CAD build for the part. Positions are in the model's coordinates, mm. Round coordinates to 2 decimals unless told otherwise and drop trailing zeros. Order: outer loops, then holes, each group sorted by start corner. A loop starts at its lowest first (then second) coordinate and runs counter-clockwise, first axis right, second up. Notation, with made-up numbers: M 33.5,80.25 L 76.5,80.25 A31 cw 76.5,111.25 Z; hole C 30.5,70.5 d4. An arc over 180 degrees is marked long. Put each result on its own line as item: value.
```python
from build123d import *

# Parameters (mm, degrees)
SKETCH_1_R      = 2.25
SKETCH_1_R_2    = 1.7
SKETCH_1_R_3    = 6
SKETCH_1_R_4    = 4.75
SKETCH_1_R_5    = 5
SKETCH_1_R_6    = 1.69491354
EXTRUDE_1_DEPTH = 2


with BuildPart() as part:
    # 草图1 → 凸台-拉伸1 (new body)
    with BuildSketch(Plane(origin=(0, 0, 0), x_dir=(1, 0, 0), z_dir=(0, 1, 0))):
        Polygon((-41.878679656, -46.121320344), (42.121320344, -46.121320344), (44.23849367, -43.995861074), (44.23849367, 44.004138926), (42.249509012, 46.250010702), (-42.015698652, 46.250010702), (-44, 44), (-44, -44), align=None)
        with Locations(Location((-15.25, -15.25, 0), (0, 0, 270))):
            Circle(SKETCH_1_R, mode=Mode.SUBTRACT)
        with Locations(Location((-15.25, 15.25, 0), (0, 0, 270))):
            Circle(SKETCH_1_R, mode=Mode.SUBTRACT)
        with Locations(Location((15.25, -15.25, 0), (0, 0, 270))):
            Circle(SKETCH_1_R, mode=Mode.SUBTRACT)
        with Locations(Location((15.25, 15.25, 0), (0, 0, 270))):
            Circle(SKETCH_1_R, mode=Mode.SUBTRACT)
        with Locations(Location((-24, -33, 0), (0, 0, 270))):
            Circle(SKETCH_1_R_2, mode=Mode.SUBTRACT)
        with Locations(Location((20, 0, 0), (0, 0, 270))):
            Circle(SKETCH_1_R_3, mode=Mode.SUBTRACT)
        with Locations(Location((-20, 0, 0), (0, 0, 270))):
            Circle(SKETCH_1_R_4, mode=Mode.SUBTRACT)
        with Locations(Location((0, 26, 0), (0, 0, 270))):
            Circle(SKETCH_1_R_5, mode=Mode.SUBTRACT)
        with Locations(Location((0, -26, 0), (0, 0, 270))):
            Circle(SKETCH_1_R_5, mode=Mode.SUBTRACT)
        with Locations(Location((-30.40559154, -40.30508646, 0), (0, 0, 270))):
            Circle(SKETCH_1_R_2, mode=Mode.SUBTRACT)
        with Locations(Location((-30.40559154, 40.30508646, 0), (0, 0, 270))):
            Circle(SKETCH_1_R_2, mode=Mode.SUBTRACT)
        with Locations(Location((-40.30508646, 30.40559154, 0), (0, 0, 270))):
            Circle(SKETCH_1_R_2, mode=Mode.SUBTRACT)
        with Locations(Location((30.40559154, -40.30508646, 0), (0, 0, 270))):
            Circle(SKETCH_1_R_2, mode=Mode.SUBTRACT)
        with Locations(Location((40.30508646, -31, 0), (0, 0, 270))):
            Circle(SKETCH_1_R_6, mode=Mode.SUBTRACT)
        with Locations(Location((40.30508646, 30.40559154, 0), (0, 0, 270))):
            Circle(SKETCH_1_R_6, mode=Mode.SUBTRACT)
        with Locations(Location((30.40559154, 40.30508646, 0), (0, 0, 270))):
            Circle(SKETCH_1_R_2, mode=Mode.SUBTRACT)
        with Locations(Location((-40.30508646, -30.40559154, 0), (0, 0, 90))):
            Circle(SKETCH_1_R_2, mode=Mode.SUBTRACT)
        with Locations(Location((24, -33, 0), (0, 0, 90))):
            Circle(SKETCH_1_R_2, mode=Mode.SUBTRACT)
        with Locations(Location((24, 33, 0), (0, 0, 270))):
            Circle(SKETCH_1_R_2, mode=Mode.SUBTRACT)
        with Locations(Location((-24, 33, 0), (0, 0, 90))):
            Circle(SKETCH_1_R_2, mode=Mode.SUBTRACT)
    extrude(amount=EXTRUDE_1_DEPTH)


solid = part.part
```
Item 1: Band-saw the part on D-D on y = 0.7. State how many separate pieces and enclosed holes the cut face has, and give its area (3 significant figures).
Answers below:
separate pieces: 1
enclosed holes: 20
area: 7,630 mm²
Item 2: Band-saw the part on B-B on x = 20. Give the cut face in (y, z).
Answers below:
outline: M 0,-46.25 L 2,-46.25 L 2,-6 L 0,-6 Z; M 0,6 L 2,6 L 2,46.12 L 0,46.12 Z
Item 3: Mould opens along Z. For faces 1 (the cylindrical face through (21.802, 0.986, 5.723)), 2 (the flat face through (43.17, 0.99, 45.07)), 3 (the flat face through (-42.994, 0.986, -45.141)), 4 (the cylindrical face through (25.433, 0.986, -32.086)) say: pulls with the +Z half, pulls with the -Z half, needs draft (parallel to the pull), parting line crosses it, or undercut.
Answers below:
face 1: undercut
face 2: pulls with the +Z half
face 3: pulls with the -Z half
face 4: undercut
Item 4: Band-saw the part on A-A on x = 0. Give the cut face in (y, z), and give its area (3 significant figures).
Answers below:
outline: M 0,-46.25 L 2,-46.25 L 2,-31 L 0,-31 Z; M 0,-21 L 2,-21 L 2,21 L 0,21 Z; M 0,31 L 2,31 L 2,46.12 L 0,46.12 Z
area: 145 mm²
Item 5: Probe line 1 along X through (y, z) = (0.6, 0); line 2 along X through (y, z) = (1.15, 40); line 3 along X through (y, z) = (1.5, -25.5). List the from-to ranges inside material, lowest first. Write a range as [from, to].
Answers below:
line 1: [-44, -24.75], [-15.25, 14], [26, 44.24]
line 2: [-44, -32.08], [-28.73, 28.73], [32.08, 44.24]
line 3: [-44, -4.97], [4.97, 44.24]
Item 6: Band-saw the part on C-C on z = 26. Give the cut face in (x, y), and give its area (3 significant figures).
Answers below:
outline: M -44,0 L -5,0 L -5,2 L -44,2 Z; M 5,0 L 44.24,0 L 44.24,2 L 5,2 Z
area: 156 mm²
Item 7: Pin check, flat tip, straight feed: P1, Ø2, axis at x = 40.31, z = -30.41, coming from the -Y side. Stop position of the tip, or through.
Answers below:
P1: through
